Part model, mm, in its own coordinate system. A direction names the side the tool comes from. Coordinates: 2 decimals unless noted, no trailing zeros. Order: outer loops, then holes, each group sorted by start corner. A loop starts at its lowest first (then second) coordinate and runs counter-clockwise, first axis right, second up.
1) Pin check, flat tips, straight feed: pin 1 Ø12 at (x, z) = (1, 6) entering from -Y; pin 2 Ø3 at (y, z) = (2, 22) entering from +X; pin 3 Ø1.5 at (x, y) = (-73.5, 6) entering from +Z; pin 4 Ø1.5 at (x, y) = (-69, 3.5) entering from -Z. Stop position of each tip, or through.
2) Mould opens along Z. For faces 1 (the flat face through (-6.94, 4.93, -52.47)), 2 (the flat face through (-5, 0, 5)), 3 (the cylindrical face through (13.281, 4.93, -63.243)), 4 (the flat face through (-6.371, 4.93, -15.705)) say: +Z half, -Z half, draft (parallel to the pull), parting line (faces both ways), or undercut.
3) Tool access for faces 5 (the cylindrical face through (-8.53, 4.93, -37.22)), 6 (the cylindrical face through (-7.7, 4.93, -36.65)), 7 (the flat face through (-33.52, 4.93, -42.47)): list every direction of +Z, -Z, +X, -X, +Y, -Y with a clear straight run to the whole face (end or side of a thin tool).
4) Wall check: L1, parallel to X at y = 5.25, z = -56; L2, parallel to X at y = 1.25, z = 31.5; L3, parallel to Z at x = -30, y = 5.5. Give the ranges that are in metal, low to high.
5) Cut at C-C (y = 3). List the corners of the cut face in (x, z).
6) Cut at A-A (x = -85). List the corners of the cut face in (y, z), and give its area (3 significant figures).
7) Cut at B-B (z = -53). List the corners of the cut face in (x, y).
```python
from build123d import *

# Parameters (mm, degrees)
BOSS_EXTRUDE1_DEPTH = 10


with BuildPart() as part:
    # Sketch1 → Boss-Extrude1 (new body)
    with BuildSketch(Plane(origin=(0, 0, 0), x_dir=(1, 0, 0), z_dir=(0, 1, 0))):
        with BuildLine():
            Line((-3.197802304, 60.450073138), (-10.78557004, 44.267462694))
            ThreePointArc((-10.78557004, 44.267462694), (-12.997646781, 41.849514237), (-16.192346026, 41.118997306))
            Line((-16.192346026, 41.118997306), (-51.345713088, 43.856493285))
            ThreePointArc((-51.345713088, 43.856493285), (-90.906449046, -43.828164288), (-4.486759028, -1.575493597))
            Line((-4.486759028, -1.575493597), (-8.309742442, 33.476437845))
            ThreePointArc((-8.309742442, 33.476437845), (-7.678341525, 36.692194542), (-5.329937086, 38.977966806))
            Line((-5.329937086, 38.977966806), (10.610355689, 47.062406568))
            ThreePointArc((10.610355689, 47.062406568), (13.089481768, 63.434160758), (-3.197802304, 60.450073138))
        make_face()
        with BuildLine():
            ThreePointArc((-5.480863845, -1.683916901), (-90.210358478, -43.110210305), (-51.423350976, 42.859511662))
            Line((-51.423350976, 42.859511662), (-16.269983915, 40.122015682))
            ThreePointArc((-16.269983915, 40.122015682), (-12.494430262, 40.985353873), (-9.880157749, 43.842929323))
            Line((-9.880157749, 43.842929323), (-2.292390013, 60.025539767))
            ThreePointArc((-2.292390013, 60.025539767), (12.393391201, 62.716206775), (10.158033664, 47.954261256))
            Line((10.158033664, 47.954261256), (-5.782259111, 39.869821495))
            ThreePointArc((-5.782259111, 39.869821495), (-8.557646175, 37.168454274), (-9.303847259, 33.368014541))
            Line((-9.303847259, 33.368014541), (-5.480863845, -1.683916901))
        make_face(mode=Mode.SUBTRACT)
    extrude(amount=BOSS_EXTRUDE1_DEPTH)


solid = part.part
```
Geometry check:
1. pin 1: stops at y = 0
1. pin 2: stops at x = -5.97
1. pin 3: stops at z = 55.18
1. pin 4: stops at z = -42.35
2. face 1: -Z half
2. face 2: draft
2. face 3: parting line
2. face 4: undercut
3. face 5: +Y, -Y
3. face 6: +X, +Y, -Y
3. face 7: -Z, +Y, -Y
4. L1: x = -5.28 to -4.18, 15.18 to 16.18
4. L2: x = -100.26 to -99.12, -11.51 to -10.37
4. L3: z = -42.19 to -41.19, 50.39 to 51.54
5. outline: (-51.35, -43.86) - (-16.19, -41.12) arc R5.5 cw to (-10.79, -44.27) - (-3.2, -60.45) arc R10.17 ccw (long way) to (10.61, -47.06) - (-5.33, -38.98) arc R5.5 cw to (-8.31, -33.48) - (-4.49, 1.58) arc R51.13 ccw (long way) to start; hole (-51.42, -42.86) - (-16.27, -40.12) arc R6.5 cw to (-9.88, -43.84) - (-2.29, -60.03) arc R9.17 ccw (long way) to (10.16, -47.95) - (-5.78, -39.87) arc R6.5 cw to (-9.3, -33.37) - (-5.48, 1.68) arc R50.13 ccw (long way) to start
6. outline: (0, -34.51) - (10, -34.51) - (10, -33.28) - (0, -33.28) - close; (0, 47.52) - (10, 47.52) - (10, 48.75) - (0, 48.75) - close
6. area: 24.7 mm2
7. outline: (-6.69, 0) - (-5.59, 0) - (-5.59, 10) - (-6.69, 10) - close; (14.63, 0) - (15.69, 0) - (15.69, 10) - (14.63, 10) - close
